from build123d import *

# Parameters (mm, degrees)
F1_DEPTH = 159.004
F2_R     = 22.7154462009
F3_DEPTH = 25.4
F4_W     = 112.0414791829
F4_H     = 119.2157939076
F5_DEPTH = 39.37


with BuildPart() as f1:
    # F0 (on Top) → F1 (new body)
    with BuildSketch(Plane.XY):
        Polygon((-126.4487951994, 45.7677543163), (-70.34984231, -81.4194008708), (12.415018864, -61.5593157709), (46.0842102766, 11.474811472), (-27.5696720928, 63.6536478996), align=None)
    extrude(amount=F1_DEPTH)

    # F2 (on face) → F3 (cut)
    with BuildSketch(Plane.XY.offset(159.004)):
        with Locations((-50.3989383578, -16.7727395892)):
            Circle(F2_R)
    extrude(amount=-F3_DEPTH, mode=Mode.SUBTRACT)

    # F4 (on face) → F5 (cut)
    with BuildSketch(Plane(origin=(33.64399896, -15.5100948506, 0), x_dir=(0.4186597128, 0.9081431852, 0), z_dir=(0.9081431852, -0.4186597128, 0))):
        with Locations((-26.3063655135, 90.2826599777)):
            Rectangle(F4_W, F4_H)
    extrude(amount=-F5_DEPTH, mode=Mode.SUBTRACT)


solid = f1.part
Read the model definition and answer for the solid it produces. Units are mm, in the model's axes. A direction names the side the tool comes from. Round coordinates to 2 decimals unless told otherwise and drop trailing zeros. Order: outer loops, then holes, each group sorted by start corner. A loop starts at its lowest first (then second) coordinate and runs counter-clockwise, first axis right, second up.
1) The part is cut by section C-C on x = -11.5. Write down the section's boundary in (y, z).
2) Flat-ended cylindrical pins translate along their axes: pin 1 (10 mm diameter, centred on y = 9.5, z = 78.5, fed in from +X); pin 2 (22.5 mm diameter, centred on x = -49, y = -8.5, fed in from +Z); pin 3 (8 mm diameter, centred on y = -55.5, z = 55, fed in from -X). Find the tip coordinate at first contact, or state that the pin passes through.
3) The part is cut by section B-B on z = 43.5. Write down the section's boundary in (x, y), plus the area to 3 significant figures.
4) The part is cut by section D-D on y = -59. Write down the section's boundary in (x, z).
5) The mould has two halves that part along Z. Classify faces 1 (the face through (-41, -8, 0)), 2 (the face through (10, -20, 30.675)), 3 (the face through (-28.732, -9.95, 146.482)): released by +Z, released by -Z, zero draft, split by the parting line, or undercut.
6) The part is cut by section A-A on y = 25.5. Write down the section's boundary in (x, z).
7) Straight lines are drawn through the part: L1, parallel to Z at x = 6.5, y = -13; L2, parallel to X at y = 20, z = 37; L3, parallel to Z at x = -53, y = -7.5. For each, find the intervals that lie inside material, in ascending order.
8) For faces 4 (the face through (28.46, 19.6, 89.45)), 5 (the face through (-51, -16, 133.604)), 6 (the face through (29.014, -25.553, 15.123)), determine the directions among +Z, -Z, +X, -X, +Y, -Y from which every point of the face is accessible in a straight line to the end or side of a thin tool.
Resolved:
1. outline: (-67.3, 0) - (52.27, 0) - (52.27, 159) - (-67.3, 159) - (-67.3, 149.89) - (-19.4, 149.89) - (-19.4, 30.67) - (-67.3, 30.67) - close
2. pin 1: stops at x = 46.08
2. pin 2: stops at z = 133.6
2. pin 3: stops at x = -83.55
3. outline: (-126.45, 45.77) - (-70.35, -81.42) - (-36.33, -73.26) - (10.33, 27.96) - (46.08, 11.47) - (-27.57, 63.65) - close
3. area: 12,200 mm2
4. outline: (-80.24, 0) - (13.59, 0) - (13.59, 30.67) - (-29.76, 30.67) - (-29.76, 149.89) - (13.59, 149.89) - (13.59, 159) - (-80.24, 159) - close
5. face 1: released by -Z
5. face 2: undercut
5. face 3: zero draft
6. outline: (-117.51, 0) - (26.29, 0) - (26.29, 159) - (-117.51, 159) - close; hole (9.2, 30.67) - (15.66, 30.67) - (15.66, 149.89) - (9.2, 149.89) - close
7. L1: z = 0 to 30.67, 149.89 to 159
7. L2: x = -115.08 to 6.66, 27.59 to 34.05
7. L3: z = 0 to 133.6
8. face 4: -Y
8. face 5: +Z
8. face 6: +Z, -Z, +X, -Y
